Verification items for the finished model (mm, model axes). A direction names the side the tool comes from. Give positions to 0.01 mm unless a question says otherwise; leave off trailing zeros. Write each loop counter-clockwise with the first axis right and the second up, starting at its lowest first coordinate (ties: lowest second). Pieces come first, ordered by that corner, then holes. Notation, with made-up numbers: (20, -19.5) -> (67, -19.5) arc R25 ccw to (67, 12.5) -> close; hole circle Ø6 at (7.5, 16.25). An arc over 180 degrees is marked (long way). Answer as CSV lines item,"result". Start each with the question number.
1) Sectioned sample at D-D on x = -8. Record the cut outline in (y, z).
2) Gauge pin test, flat end, axial feed: pin 1 Ø0.9 at (x, y) = (12.5, 1.5) entering from +Z. Record the tip position at first contact, or that the pin passes through.
3) Material ranges on L1, parallel to X at y = 0.9, z = -33; L2, parallel to X at y = 2.2, z = 33; L3, parallel to X at y = 1.9, z = 21.5, recorded low to high.
4) Sectioned sample at C-C on z = 33. Record the cut outline in (x, y), and give its area (3 significant figures).
5) Sectioned sample at B-B on z = -33. Record the cut outline in (x, y).
6) Sectioned sample at A-A on x = -43.5. Record the cut outline in (y, z).
7) Tool access check on faces 4 (the flat face through (-72.5, 1, -1)), 5 (the flat face through (46, 1, 37)), 6 (the flat face through (28, 1, 20)). Record the directions out of +Z, -Z, +X, -X, +Y, -Y that give a thin tool (end or side, any length) a straight path to the whole face; none if there is none.
8) Mould release check, pull along Z, two halves, no side actions. Record for faces 1 (the flat face through (72.5, 1, 1)), 2 (the flat face through (10, 1, -37)), 3 (the flat face through (50, 1, 40)): released by +Z, released by -Z, zero draft, split by the parting line, or undercut.
```python
from build123d import *

# Parameters (mm, degrees)
SKETCH1_R           = 1.5
SKETCH1_W           = 3
SKETCH1_H           = 7
SKETCH1_W_2         = 4
SKETCH1_H_2         = 3
BOSS_EXTRUDE1_DEPTH = 3
SKETCH5_W           = 50
SKETCH5_H           = 8
CUT_EXTRUDE1_DEPTH  = 10


with BuildPart() as part:
    # Sketch1 → Boss-Extrude1 (new body)
    with BuildSketch(Plane(origin=(0, 0, 0), x_dir=(1, 0, 0), z_dir=(0, 1, 0))):
        Polygon((-72.5, -40), (-28, -40), (-28, 0), (28, 0), (28, -40), (72.5, -40), (72.5, 40), (-72.5, 40), align=None)
        with Locations(Location((-69.5, 33, 0), (0, 0, 270))):
            Circle(SKETCH1_R, mode=Mode.SUBTRACT)
        with Locations(Location((-43.5, 33, 0), (0, 0, 270))):
            Circle(SKETCH1_R, mode=Mode.SUBTRACT)
        with Locations(Location((-43.5, -33, 0), (0, 0, 270))):
            Circle(SKETCH1_R, mode=Mode.SUBTRACT)
        with Locations(Location((-69.5, -33, 0), (0, 0, 270))):
            Circle(SKETCH1_R, mode=Mode.SUBTRACT)
        with Locations((46, 5.5)):
            Rectangle(SKETCH1_W, SKETCH1_H, mode=Mode.SUBTRACT)
        with Locations((46, 18.5)):
            Rectangle(SKETCH1_W, SKETCH1_H, mode=Mode.SUBTRACT)
        with Locations((46, -7.5)):
            Rectangle(SKETCH1_W, SKETCH1_H, mode=Mode.SUBTRACT)
        with Locations((46, -20.5)):
            Rectangle(SKETCH1_W, SKETCH1_H, mode=Mode.SUBTRACT)
        with Locations((46, -33.5)):
            Rectangle(SKETCH1_W, SKETCH1_H, mode=Mode.SUBTRACT)
        with Locations((0, 37.5)):
            Rectangle(SKETCH1_W_2, SKETCH1_H_2, mode=Mode.SUBTRACT)
        with Locations((8, 37.5)):
            Rectangle(SKETCH1_W_2, SKETCH1_H_2, mode=Mode.SUBTRACT)
        with Locations((16, 37.5)):
            Rectangle(SKETCH1_W_2, SKETCH1_H_2, mode=Mode.SUBTRACT)
    extrude(amount=BOSS_EXTRUDE1_DEPTH)

    # Sketch5 → Cut-Extrude1 (cut)
    with BuildSketch(Plane.XZ):
        with Locations((0, -25.5)):
            Rectangle(SKETCH5_W, SKETCH5_H)
    extrude(amount=-CUT_EXTRUDE1_DEPTH, mode=Mode.SUBTRACT)


solid = part.part
```
Ans:
1,outline,"(0, -40) -> (3, -40) -> (3, -29.5) -> (0, -29.5) -> close; (0, -21.5) -> (3, -21.5) -> (3, 0) -> (0, 0) -> close"
2,pin 1,"stops at z = 0"
3,L1,"x = -72.5 to -71, -68 to -45, -42 to 72.5"
3,L2,"x = -72.5 to -71, -68 to -45, -42 to -28, 28 to 44.5, 47.5 to 72.5"
3,L3,"x = -72.5 to -28, 28 to 44.5, 47.5 to 72.5"
4,outline,"(-72.5, 0) -> (-71, 0) -> (-71, 3) -> (-72.5, 3) -> close; (-68, 0) -> (-45, 0) -> (-45, 3) -> (-68, 3) -> close; (-42, 0) -> (-28, 0) -> (-28, 3) -> (-42, 3) -> close; (28, 0) -> (44.5, 0) -> (44.5, 3) -> (28, 3) -> close; (47.5, 0) -> (72.5, 0) -> (72.5, 3) -> (47.5, 3) -> close"
4,area,"240 mm²"
5,outline,"(-72.5, 0) -> (-71, 0) -> (-71, 3) -> (-72.5, 3) -> close; (-68, 0) -> (-45, 0) -> (-45, 3) -> (-68, 3) -> close; (-42, 0) -> (72.5, 0) -> (72.5, 3) -> (-42, 3) -> close"
6,outline,"(0, -40) -> (3, -40) -> (3, -34.5) -> (0, -34.5) -> close; (0, -31.5) -> (3, -31.5) -> (3, 31.5) -> (0, 31.5) -> close; (0, 34.5) -> (3, 34.5) -> (3, 40) -> (0, 40) -> close"
7,face 4,"+Z, -Z, -X, +Y, -Y"
7,face 5,"+Y, -Y"
7,face 6,"+Z, +Y, -Y"
8,face 1,"zero draft"
8,face 2,"undercut"
8,face 3,"released by +Z"
